Part model, mm, in its own coordinate system. Face numbers are marked on the shaded views. Round coordinates to 2 decimals unless told otherwise and drop trailing zeros. Order: outer loops, then holes, each group sorted by start corner. A loop starts at its lowest first (then second) coordinate and runs counter-clockwise, first axis right, second up. Notation, with made-up numbers: M 40,54.5 L 96,54.5 A16 ccw 96,72.5 Z; hole C 6,36 d5. An arc over 180 degrees is marked long. Write each question's results on one line, items separated by ' | '. Start each with the question number.
1. Drop flat-ended pins along their axis: pin 1 Ø3 at (x, y) = (35.4, 6.57) entering from +Z; pin 2 Ø2 at (x, z) = (-17.5, 1) entering from -Y; pin 3 Ø2 at (x, z) = (10, 1) entering from -Y. Give the stop position or say it passes through.
2. Band-saw the part on A-A, the plane x = 0. List the corners of the cut face in (y, z).
3. Band-saw the part on D-D, the plane y = -30. List the corners of the cut face in (x, z).
4. Probe L1, parallel to Y at x = -11.5, z = 2.45; L2, parallel to Y at x = -12, z = 0.8; L3, parallel to X at y = -7, z = 2.85 (3 decimals). List the from-to ranges inside material, lowest first. Write a range as [from, to].
5. Band-saw the part on C-C, the plane z = 4.15. List the corners of the cut face in (x, y), then the cut area to 3 significant figures.
6. Two-plate mould, pull along X, no slides. Class the marked faces 1, 2 and 3: +X half, -X half, draft (parallel to the pull), parting line (faces both ways), or undercut.
```python
from build123d import *

# Parameters (mm, degrees)
SKETCH1_R           = 40
BOSS_EXTRUDE1_DEPTH = 5
SKETCH2_R           = 20
CUT_EXTRUDE1_DEPTH  = 6
SKETCH3_R           = 1.7
CUT_EXTRUDE2_DEPTH  = 6


with BuildPart() as part:
    # Sketch1 → Boss-Extrude1 (new body)
    with BuildSketch(Plane.XY):
        Circle(SKETCH1_R)
    extrude(amount=BOSS_EXTRUDE1_DEPTH)

    # Sketch2 → Cut-Extrude1 (cut, through all)
    with BuildSketch(Plane(origin=(0, 0, 0), x_dir=(-1, 0, 0), z_dir=(0, 0, -1))):
        Circle(SKETCH2_R)
    extrude(amount=-CUT_EXTRUDE1_DEPTH, mode=Mode.SUBTRACT)

    # Sketch3 → Cut-Extrude2 (cut, through all)
    with BuildSketch(Plane.XY.offset(5)):
        with Locations((12.009212016, 33.937867151)):
            Circle(SKETCH3_R)
        with Locations((35.395661111, 6.56865089)):
            Circle(SKETCH3_R)
        with Locations((23.386449095, -27.369216261)):
            Circle(SKETCH3_R)
        with Locations((-12.009212016, -33.937867151)):
            Circle(SKETCH3_R)
        with Locations((-35.395661111, -6.56865089)):
            Circle(SKETCH3_R)
        with Locations((-23.386449095, 27.369216261)):
            Circle(SKETCH3_R)
    extrude(amount=-CUT_EXTRUDE2_DEPTH, mode=Mode.SUBTRACT)


solid = part.part
```
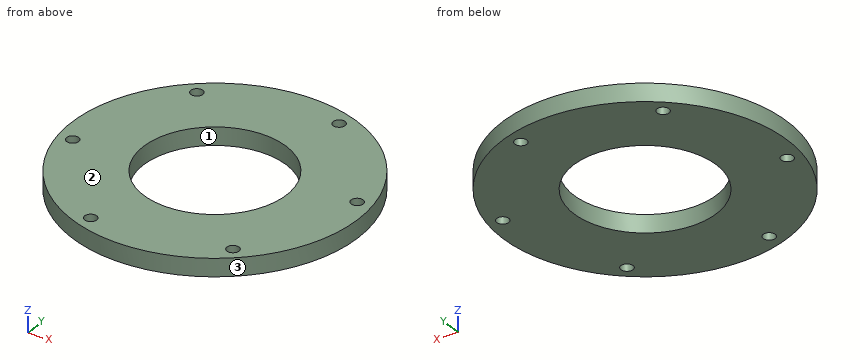
Solution:
1) pin 1: through | pin 2: y = -36.44 | pin 3: y = -38.97
2) outline: M -40,0 L -20,0 L -20,5 L -40,5 Z; M 20,0 L 40,0 L 40,5 L 20,5 Z
3) outline: M -26.46,0 L 26.46,0 L 26.46,5 L -26.46,5 Z
4) L1: [-38.31, -35.56], [-32.32, -16.36], [16.36, 38.31] | L2: [-38.16, -35.64], [-32.24, -16], [16, 38.16] | L3: [-39.383, -37.04], [-33.751, -18.735], [18.735, 39.383]
5) outline: C 0,0 d80; hole C -35.4,-6.57 d3.4; hole C -23.39,27.37 d3.4; hole C 0,0 d40; hole C -12.01,-33.94 d3.4; hole C 12.01,33.94 d3.4; hole C 23.39,-27.37 d3.4; hole C 35.4,6.57 d3.4 | area: 3,720 mm^2
6) face 1: undercut | face 2: draft | face 3: parting line
